```python
from build123d import *

# Parameters (mm, degrees)
SKETCH007_W                     = 85
SKETCH007_H                     = 50
PAD006_DEPTH                    = 6.5
SKETCH008_W                     = 81.5
SKETCH008_H                     = 46.5
POCKET_DEPTH                    = 4.501
SKETCH010_W                     = 9
SKETCH010_H                     = 9
PAD007_DEPTH                    = 4.3
SKETCH010_MIRRORED002_2_W       = 9
SKETCH010_MIRRORED002_2_H       = 9
PAD007_MIRRORED002_2_DEPTH      = 4.3
CYLINDER001_R                   = 2
CYLINDER001_DEPTH               = 10
CYLINDER001_MIRRORED004_2_R     = 2
CYLINDER001_MIRRORED004_2_DEPTH = 10
SKETCH017_W                     = 4.302639
SKETCH017_H                     = 32
POCKET006_DEPTH                 = 5
CHAMFER_SIZE                    = 1.5


with BuildPart() as part:
    # Sketch007 → Pad006 (new body)
    with BuildSketch(Plane.XY):
        Rectangle(SKETCH007_W, SKETCH007_H)
    extrude(amount=PAD006_DEPTH)

    # Sketch008 → Pocket (cut, through all)
    with BuildSketch(Plane.XY.offset(2)):
        Rectangle(SKETCH008_W, SKETCH008_H)
    extrude(amount=POCKET_DEPTH, mode=Mode.SUBTRACT)

    # Sketch010 → Pad007 (join)
    with BuildSketch(Plane.XY):
        with Locations((-38, -20.5)):
            Rectangle(SKETCH010_W, SKETCH010_H)
    pad007 = extrude(amount=PAD007_DEPTH)

    # Sketch010 Mirrored002 2 → Pad007 Mirrored002 2 (add)
    with BuildSketch(Plane(origin=(0, 0, 0), x_dir=(-1, 0, 0), z_dir=(0, 0, -1))):
        with Locations((-38, -20.5)):
            Rectangle(SKETCH010_MIRRORED002_2_W, SKETCH010_MIRRORED002_2_H)
    pad007_mirrored002_2 = extrude(amount=-PAD007_MIRRORED002_2_DEPTH)

    # Mirrored003: Pad007, Pad007 Mirrored002 2 across Sketch010 H_Axis
    add(pad007.mirror(Plane.ZX))
    add(pad007_mirrored002_2.mirror(Plane.ZX))

    # Cylinder001 → Cylinder001 (cut)
    with BuildSketch(Plane(origin=(-37, -19.5, 0), x_dir=(1, 0, 0), z_dir=(0, 0, 1))):
        Circle(CYLINDER001_R)
    cylinder001 = extrude(amount=CYLINDER001_DEPTH, mode=Mode.SUBTRACT)

    # Cylinder001 Mirrored004 2 → Cylinder001 Mirrored004 2 (cut)
    with BuildSketch(Plane(origin=(37, -19.5, 0), x_dir=(-1, 0, 0), z_dir=(0, 0, -1))):
        Circle(CYLINDER001_MIRRORED004_2_R)
    cylinder001_mirrored004_2 = extrude(amount=-CYLINDER001_MIRRORED004_2_DEPTH, mode=Mode.SUBTRACT)

    # Mirrored005: Cylinder001, Cylinder001 Mirrored004 2 across XZ
    add(cylinder001.mirror(Plane.XZ), mode=Mode.SUBTRACT)
    add(cylinder001_mirrored004_2.mirror(Plane.XZ), mode=Mode.SUBTRACT)

    # Sketch017 → Pocket006 (cut)
    with BuildSketch(Plane.XY.offset(6.5)):
        with Locations((-41.55937, 0)):
            Rectangle(SKETCH017_W, SKETCH017_H)
    extrude(amount=POCKET006_DEPTH, mode=Mode.SUBTRACT)

    # Chamfer
    chamfer_edges = [part.edges().sort_by_distance(p)[0] for p in [
        (-39, -19.5, 0),
        (-39, 19.5, 0),
    ]]
    chamfer(chamfer_edges, length=CHAMFER_SIZE)


solid = part.part
```
Source: CAD feature listing. Evaluate the final solid. Frame: model axes, mm. A direction names the side the tool comes from. Round coordinates to 2 decimals unless told otherwise and drop trailing zeros. Loops run counter-clockwise (first coordinate to the right, second up) from the corner with the lowest first, then second, coordinate; pieces in that order, holes last.
1. Section query B-B on y = 19.5. Output: boundary loops of the cut face in (x, z).
2. Section query C-C on x = -37. Output: boundary loops of the cut face in (y, z), and give its area (3 significant figures).
3. Section query D-D on x = 14. Output: boundary loops of the cut face in (y, z), and give its area (3 significant figures).
4. Ray query, L1, parallel to X at y = 19.5, z = 3.2; L2, parallel to Y at x = -37, z = 3.75; L3, parallel to X at y = 1.5, z = 2.75. Return the intervals inside material, ascending.
5. Mould query, pull axis X, two halves, no side actions, for faces 1 (the flat face through (33.5, 20, 3)), 2 (the flat face through (-13, -24, 6.5)), 3 (the flat face through (42.5, 0, 3)). Classes: released by +X, released by -X, zero draft, split by the parting line, or undercut.
6. Access query for faces 4 (the flat face through (40.75, 0, 4)), 5 (the cylindrical face through (-37.26, 17.517, 2.88)). Directions: +Z, -Z, +X, -X, +Y, -Y. A direction counts if a zero-diameter tool reaches every point of the face in a straight line with its end or side. Return the directions, or none.
7. Contact query for flat-ended pins moving along their axis: pin 1 (8 mm diameter, centred on x = -37, y = 18.5, fed in from +Z); pin 2 (4 mm diameter, centred on x = -6, y = -11.5, fed in from +Z); pin 3 (6 mm diameter, centred on x = 37, y = -18.5, fed in from +Z); pin 4 (4.5 mm diameter, centred on x = -37, y = 19.5, fed in from -Z). Output: stop coordinate, or through.
8. Section query A-A on z = 3.5. Output: boundary loops of the cut face in (x, y), and give its area (3 significant figures).
Answers below:
1. outline: (-42.5, 0) - (-40.5, 0) - (-39, 1.5) - (-39, 4.3) - (-40.75, 4.3) - (-40.75, 6.5) - (-42.5, 6.5) - close; (-35, 1.5) - (-33.5, 0) - (35, 0) - (35, 4.3) - (33.5, 4.3) - (33.5, 2) - (-33.5, 2) - (-33.5, 4.3) - (-35, 4.3) - close; (39, 0) - (42.5, 0) - (42.5, 6.5) - (40.75, 6.5) - (40.75, 4.3) - (39, 4.3) - close
2. outline: (-25, 0) - (-23, 0) - (-21.5, 1.5) - (-21.5, 4.3) - (-23.25, 4.3) - (-23.25, 6.5) - (-25, 6.5) - close; (-17.5, 1.5) - (-16, 0) - (16, 0) - (17.5, 1.5) - (17.5, 4.3) - (16, 4.3) - (16, 2) - (-16, 2) - (-16, 4.3) - (-17.5, 4.3) - close; (21.5, 1.5) - (23, 0) - (25, 0) - (25, 6.5) - (23.25, 6.5) - (23.25, 4.3) - (21.5, 4.3) - close
2. area: 110 mm2
3. outline: (-25, 0) - (25, 0) - (25, 6.5) - (23.25, 6.5) - (23.25, 2) - (-23.25, 2) - (-23.25, 6.5) - (-25, 6.5) - close
3. area: 116 mm2
4. L1: x = -42.5 to -39, -35 to -33.5, 33.5 to 35, 39 to 42.5
4. L2: y = -25 to -21.5, -17.5 to -16, 16 to 17.5, 21.5 to 25
4. L3: x = -42.5 to -40.75, 40.75 to 42.5
5. face 1: undercut
5. face 2: zero draft
5. face 3: released by +X
6. face 4: +Z
6. face 5: +Z, -Z
7. pin 1: stops at z = 6.5
7. pin 2: stops at z = 2
7. pin 3: stops at z = 4.3
7. pin 4: stops at z = 1.25
8. outline: (-42.5, -25) - (42.5, -25) - (42.5, 25) - (-42.5, 25) - close; hole (-40.75, -16) - (-33.5, -16) - (-33.5, -23.25) - (33.5, -23.25) - (33.5, -16) - (40.75, -16) - (40.75, 16) - (33.5, 16) - (33.5, 23.25) - (-33.5, 23.25) - (-33.5, 16) - (-40.75, 16) - close; hole circle Ø4 at (-37, -19.5); hole circle Ø4 at (-37, 19.5); hole circle Ø4 at (37, -19.5); hole circle Ø4 at (37, 19.5)
8. area: 620 mm2
